```python
from build123d import *

# Parameters (mm, degrees)
F0_R           = 1.016
F1_DEPTH       = 17.526
F3_START       = -25.4
F3_DEPTH       = 40.641
F4_R           = 3.81
F5_DEPTH       = 6.35
F7_D           = 2.032
F7_CSINK_D     = 3.175
F7_CSINK_ANGLE = 82


with BuildPart() as f1:
    # F0 (on Top) → F1 (new body)
    with BuildSketch(Plane.XY):
        with BuildLine():
            Line((15.24, 40.64), (0, 40.64))
            Line((0, 40.64), (-15.24, 40.64))
            Line((-15.24, 40.64), (-15.24, -13.97))
            Line((-15.24, -13.97), (-7.7384455959, -27.2359067358))
            ThreePointArc((-7.7384455959, -27.2359067358), (-2.2624454306, -14.2627073637), (8.89, -22.86))
            ThreePointArc((8.89, -22.86), (8.5972926363, -25.1224454306), (7.7384455959, -27.2359067358))
            Line((7.7384455959, -27.2359067358), (15.24, -13.97))
            Line((15.24, -13.97), (15.24, 40.64))
        make_face()
        with Locations((-5.4991, -13.97)):
            Circle(F0_R, mode=Mode.SUBTRACT)
        with Locations((5.4991, -13.97)):
            Circle(F0_R, mode=Mode.SUBTRACT)
        with Locations((-5.4991, 34.036)):
            Circle(F0_R, mode=Mode.SUBTRACT)
        Polygon((10.16, -10.16), (0, -10.16), (-10.16, -10.16), (-10.16, 30.48), (0, 30.48), (10.16, 30.48), align=None, mode=Mode.SUBTRACT)
        with Locations((5.4991, 34.036)):
            Circle(F0_R, mode=Mode.SUBTRACT)
        with BuildLine():
            ThreePointArc((8.89, -22.86), (-2.2624454306, -14.2627073637), (-7.7384455959, -27.2359067358))
            ThreePointArc((-7.7384455959, -27.2359067358), (0, -31.75), (7.7384455959, -27.2359067358))
            ThreePointArc((7.7384455959, -27.2359067358), (8.5972926363, -25.1224454306), (8.89, -22.86))
        make_face()
    extrude(amount=F1_DEPTH)

    # F2 (on Right) → F3 (intersect)
    with BuildSketch(Plane.YZ.offset(F3_START)):
        Polygon((-31.7592067564, 5.08), (-31.7592067564, 0), (-16.4593220198, 0), (-16.4593220198, 3.556), (-10.0653828302, 11.176), (41.7786614893, 11.176), (41.7786614893, 17.526), (-21.3157727468, 17.526), align=None)
    extrude(amount=F3_DEPTH, mode=Mode.INTERSECT)

    # F4 (on Top) → F5 (join)
    with BuildSketch(Plane.XY):
        with Locations((0, -22.86)):
            Circle(F4_R)
    extrude(amount=-F5_DEPTH)

    # F7 (through all)
    with Locations(Plane(origin=(0, 0, -6.35), x_dir=(1, 0, 0), z_dir=(0, 0, -1))):
        with Locations((0, 22.86)):
            CounterSinkHole(F7_D / 2, F7_CSINK_D / 2, counter_sink_angle=F7_CSINK_ANGLE)


solid = f1.part
```
Could you check a few things on this model? Use its own coordinates, in mm. A direction names the side the tool comes from. Coordinates: 2 decimals unless noted, no trailing zeros. Order: outer loops, then holes, each group sorted by start corner. A loop starts at its lowest first (then second) coordinate and runs counter-clockwise, first axis right, second up. Notation, with made-up numbers: M 86,70.25 L 113,70.25 A21 ccw 113,101.25 Z; hole C 65,46 d7. An arc over 180 degrees is marked long. Use a Markdown table: item, result. Add a question column.
Q1. I want a section at B-B on x = 0. List the corners of the cut face in (y, z) for me.
Q2. Which directions (+Z, -Z, +X, -X, +Y, -Y) give clear straight access to the entire face, cutting with the end or side of a thin tool? Please do faces 1 (the cylindrical face through (-0.83, -26.58, -3.13)), 2 (the flat face through (-10.16, 10, 14)), 3 (the flat face through (2, -23, -6.35)).
Q3. We'd pull the mould along X, two halves only. Please class faces 4 (the flat face through (15.24, 13, 14)), 5 (the flat face through (0, -16.459, 2)), 6 (the cylindrical face through (5.279, -14.962, 11.319)): pulls with the +X half, pulls with the -X half, needs draft (parallel to the pull), parting line crosses it, or undercut.
Q4. If I drill on L1, parallel to Y at x = 5.5, z = 12.25; L2, parallel to Z at x = 2, y = 36; L3, parallel to X at y = 14.5, z = 13.5, over which ranges is the centre line in solid material (lowest first)?
Q5. I want a section at D-D on x = 8.5. List the corners of the cut face in (y, z) for me, then the cut area to 3 significant figures.
Q6. I want a section at A-A on y = 4. List the corners of the cut face in (x, z) for me, then the cut area to 3 significant figures.
Q7. I want a section at C-C on z = -1.5. List the corners of the cut face in (x, y) for me.
Q8. I'm going to push flat-ended pins straight in: pin 1 (4 mm diameter, centred on x = -9, z = 6, fed in from +Y); pin 2 (5 mm diameter, centred on x = -5, z = 13.5, fed in from -Y); pin 3 (6 mm diameter, centred on x = 5.5, y = 13, fed in from +Z); pin 4 (8 mm diameter, centred on y = -20, z = 8.5, fed in from +X). Where does each tip first touch, or does it pass through?
Checked values:
| question | item | result |
|---|---|---|
| 1 | outline | M -31.75,0 L -26.67,0 L -26.67,-6.35 L -24.45,-6.35 L -23.88,-5.69 L -23.88,14.47 L -31.75,5.09 Z; M -21.84,-5.69 L -21.27,-6.35 L -19.05,-6.35 L -19.05,0 L -16.46,0 L -16.46,3.56 L -10.16,11.06 L -10.16,17.53 L -21.32,17.53 L -21.84,16.9 Z; M 30.48,11.18 L 40.64,11.18 L 40.64,17.53 L 30.48,17.53 Z |
| 2 | face 1 | -Z |
| 2 | face 2 | +Z, -Z |
| 2 | face 3 | -Z, +X, -X, +Y, -Y |
| 3 | face 4 | pulls with the +X half |
| 3 | face 5 | needs draft |
| 3 | face 6 | undercut |
| 4 | L1 | -25.74 to -14.99, -12.95 to -10.16, 30.48 to 33.02, 35.05 to 40.64 |
| 4 | L2 | 11.18 to 17.53 |
| 4 | L3 | -15.24 to -10.16, 10.16 to 15.24 |
| 5 | outline | M -25.89,0 L -16.46,0 L -16.46,3.56 L -10.16,11.06 L -10.16,17.53 L -21.32,17.53 L -25.89,12.08 Z; M 30.48,11.18 L 40.64,11.18 L 40.64,17.53 L 30.48,17.53 Z |
| 5 | area | 282 mm² |
| 6 | outline | M -15.24,11.18 L -10.16,11.18 L -10.16,17.53 L -15.24,17.53 Z; M 10.16,11.18 L 15.24,11.18 L 15.24,17.53 L 10.16,17.53 Z |
| 6 | area | 64.5 mm² |
| 7 | outline | C 0,-22.86 d7.62; hole C 0,-22.86 d2.03 |
| 8 | pin 1 | y = -12.73 |
| 8 | pin 2 | y = -26.79 |
| 8 | pin 3 | through |
| 8 | pin 4 | x = 14.09 |
